Geometry check sheet. Reference: the model listing, model coordinates, mm. Face numbers are marked on the shaded views. A direction names the side the tool comes from. Coordinates: 2 decimals unless noted, no trailing zeros. Loops run counter-clockwise (first coordinate to the right, second up) from the corner with the lowest first, then second, coordinate; pieces in that order, holes last.
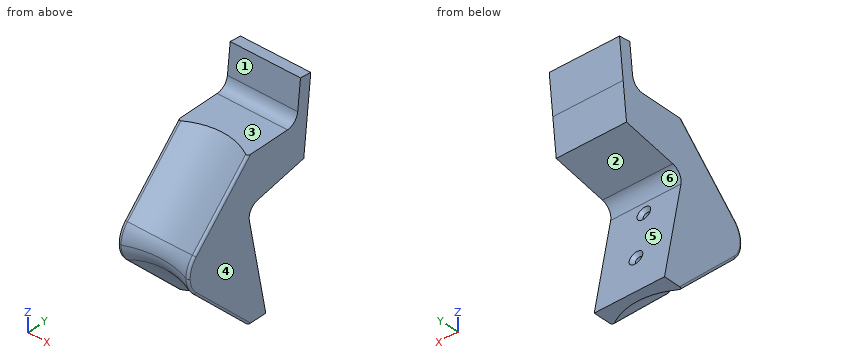
from build123d import *

# Parameters (mm, degrees)
BOSS_EXTRUDE1_DEPTH             = 9
SKETCH4_W                       = 18
SKETCH4_H                       = 44.313566923
CUT_EXTRUDE3_DEPTH              = 6
FILLET1_R                       = 0.5
CUT_EXTRUDE4_DEPTH              = 20
F_2_56_TAPPED_HOLE1_D           = 1.778
F_2_56_TAPPED_HOLE1_DEPTH       = 6.64
F_2_56_TAPPED_HOLE1_CSINK_D     = 3.4544
F_2_56_TAPPED_HOLE1_CSINK_ANGLE = 90
F_2_56_TAPPED_HOLE1_TIP         = 0.53416509
CUT_EXTRUDE5_DEPTH              = 19.0000001
BOSS_EXTRUDE2_DEPTH             = 18
FILLET2_R                       = 3


with BuildPart() as part:
    # Sketch1 → Boss-Extrude1 (new body, symmetric)
    with BuildSketch(Plane(origin=(0, 0, 0), x_dir=(0, 0, -1), z_dir=(1, 0, 0))):
        with BuildLine():
            Line((3.00520382, -3.00520382), (20, 13.98959236))
            Line((20, 13.98959236), (20, 30))
            Line((20, 30), (0, 30))
            Line((0, 30), (0, -4.25))
            ThreePointArc((0, -4.25), (1.626404588, -3.926488013), (3.00520382, -3.00520382))
        make_face()
    extrude(amount=BOSS_EXTRUDE1_DEPTH, both=True)

    # Sweep1: sweep along a path in Sketch2
    with BuildLine(Plane(origin=(0, 0, 0), x_dir=(0, 0, -1), z_dir=(1, 0, 0))) as sweep1_path:
        Line((20, 13.98959236), (3.00520382, -3.00520382))
        ThreePointArc((3.00520382, -3.00520382), (1.626404588, -3.926488013), (0, -4.25))
    # Sketch3 → Sweep1 (sweep)
    with BuildSketch(Plane.XY):
        with BuildLine():
            Line((9, -4.25), (-9, -4.25))
            Line((-9, -4.25), (-9, -6.701215317))
            ThreePointArc((-9, -6.701215317), (0, -4.65), (9, -6.701215317))
            Line((9, -6.701215317), (9, -4.25))
        make_face()
    sweep(path=sweep1_path.line)

    # Sketch4 → Cut-Extrude3 (cut)
    with BuildSketch(Plane(origin=(0, 0, -20), x_dir=(-1, 0, 0), z_dir=(0, 0, -1))):
        with Locations((0, 7.843216539)):
            Rectangle(SKETCH4_W, SKETCH4_H)
    extrude(amount=CUT_EXTRUDE3_DEPTH, mode=Mode.SUBTRACT)

    # Fillet1
    fillet1_edges = [part.edges().sort_by_distance(p)[0] for p in [
        (9, 2.89228781, -12.369237397),
        (-9, 2.89228781, -12.369237397),
        (9, -6.191115675, -2.564444079),
        (-9, -6.191115675, -2.564444079),
    ]]
    fillet(fillet1_edges, radius=FILLET1_R)

    # Mirror1: part across plane


with BuildPart() as part_1:
    add(part.part)
    add(part.part.mirror(Plane(origin=(9, 30, 0), x_dir=(1, 0, 0), z_dir=(0, 0, -1))))

    # Sketch5 → Cut-Extrude4 (cut, symmetric)
    with BuildSketch(Plane(origin=(0, 0, 0), x_dir=(0, 0, -1), z_dir=(1, 0, 0))):
        Polygon((20, 16), (-7.485561137, 10.657348129), (-11.245391787, 30), (20, 30), align=None)
    extrude(amount=CUT_EXTRUDE4_DEPTH, both=True, mode=Mode.SUBTRACT)

    # #2-56 Tapped Hole1
    with Locations(Plane(origin=(0, 11.671404902, 2.268691293), x_dir=(1, 0, 0), z_dir=(0, 0.981627183, 0.190808995))):
        with Locations((0, 12.685487595), (0, 0.685487595)):
            CounterSinkHole(F_2_56_TAPPED_HOLE1_D / 2, F_2_56_TAPPED_HOLE1_CSINK_D / 2, depth=F_2_56_TAPPED_HOLE1_DEPTH, counter_sink_angle=F_2_56_TAPPED_HOLE1_CSINK_ANGLE)
            with Locations((0, 0, -(F_2_56_TAPPED_HOLE1_DEPTH + F_2_56_TAPPED_HOLE1_TIP / 2))):  # 118° drill point
                Cone(0, F_2_56_TAPPED_HOLE1_D / 2, F_2_56_TAPPED_HOLE1_TIP, mode=Mode.SUBTRACT)

    # Sketch8 → Cut-Extrude5 (cut, through all)
    with BuildSketch(Plane.ZY.offset(9)):
        Polygon((10.6659344, 27.018950173), (20, 28), (20, 30), (11.245391787, 30), align=None)
    extrude(amount=-CUT_EXTRUDE5_DEPTH, mode=Mode.SUBTRACT)

    # Sketch10 → Boss-Extrude2 (add)
    with BuildSketch(Plane.ZY.offset(9)):
        Polygon((20, 28), (29.945218954, 29.045284633), (30.258804343, 26.061718947), (20, 24.983475161), align=None)
    extrude(amount=-BOSS_EXTRUDE2_DEPTH)

    # Fillet2
    fillet2_edges = [part_1.edges().sort_by_distance(p)[0] for p in [
        (0, 10.657348129, 7.485561137),
        (0, 24.983475161, 20),
    ]]
    fillet(fillet2_edges, radius=FILLET2_R)


solid = part_1.part
(1) Sectioned sample at B-B on x = -5. Record the cut outline in (y, z).
Findings:
outline: (-3.72, -3.72) - (12.56, -20) - (16, -20) - (11.23, 4.54) arc R3 cw to (13.6, 8.06) - (27.02, 10.67) - (29.05, 29.95) - (26.06, 30.26) - (25.27, 22.69) arc R3 cw to (22.28, 20) - (12.56, 20) - (-3.72, 3.72) arc R5.26 ccw to start
(2) Scan lines: L1, parallel to X at y = 11.5, z = -10; L2, parallel to Y at x = -5, z = 20.5; L3, parallel to Z at x = -2.5, y = 9.5. Record each from-to range of solid material in increasing order.
Findings:
L1: x = -9 to -0.58, 0.58 to 9
L2: y = 23.94 to 28.05
L3: z = -16.29 to 16.29
(3) Access from +Z, -Z, +X, -X, +Y, -Y to the whole of each face (thin tool, end or side, straight path). Record for the marked faces 1 and 2.
Findings:
face 1: +Z, +X, -X, -Y
face 2: +X, -X, +Y
(4) Sectioned sample at A-A on x = 7. Record the cut outline in (y, z), and give its area (3 significant figures).
Findings:
outline: (-4.15, -4.15) - (11.71, -20) - (16, -20) - (11.23, 4.54) arc R3 cw to (13.6, 8.06) - (27.02, 10.67) - (29.05, 29.95) - (26.06, 30.26) - (25.27, 22.69) arc R3 cw to (22.28, 20) - (11.71, 20) - (-4.15, 4.15) arc R5.87 ccw to start
area: 641 mm2
(5) Gauge pin test, flat ends, axial feed: pin 1 Ø9 at (x, y) = (0.5, 18) entering from +Z; pin 2 Ø1.5 at (x, y) = (-1, 5) entering from -Z; pin 3 Ø5 at (x, y) = (2.5, 2.5) entering from +Z. Record the tip position at first contact, or that the pin passes through.
Findings:
pin 1: stops at z = 20.01
pin 2: stops at z = -12.36
pin 3: stops at z = 11.83
(6) Draft check along Z on the marked faces 3, 4, 5 and 6. Enter one of: +Z half, -Z half, draft (parallel to the pull), parting line (faces both ways), or undercut.
Findings:
face 3: +Z half
face 4: draft
face 5: undercut
face 6: undercut
